```python
from build123d import *

# Parameters (mm, degrees)
SKETCH1_R      = 18
GEARBOX_DEPTH  = 42.5
SKETCH2_R      = 17
MOTOR_DEPTH    = 44.5
SKETCH3_R      = 11
PLATFORM_DEPTH = 2
SKETCH4_R      = 1.5
SCREWS_DEPTH   = 5


with BuildPart() as part:
    # Sketch1 → Gearbox (new body)
    with BuildSketch(Plane.XY):
        Circle(SKETCH1_R)
    extrude(amount=GEARBOX_DEPTH)

    # Sketch2 → Motor (add)
    with BuildSketch(Plane.XY.offset(42.5)):
        Circle(SKETCH2_R)
    extrude(amount=MOTOR_DEPTH)

    # Sketch3 → Platform (add)
    with BuildSketch(Plane(origin=(0, 0, 0), x_dir=(-1, 0, 0), z_dir=(0, 0, -1))):
        Circle(SKETCH3_R)
    extrude(amount=PLATFORM_DEPTH)

    # Sketch4 → Screws (cut)
    with BuildSketch(Plane(origin=(0, 0, 0), x_dir=(-1, 0, 0), z_dir=(0, 0, -1))):
        with Locations((0, 14)):
            Circle(SKETCH4_R)
        with Locations((14, 0)):
            Circle(SKETCH4_R)
        with Locations((0, -14)):
            Circle(SKETCH4_R)
        with Locations((-14, 0)):
            Circle(SKETCH4_R)
    extrude(amount=-SCREWS_DEPTH, mode=Mode.SUBTRACT)


solid = part.part
```
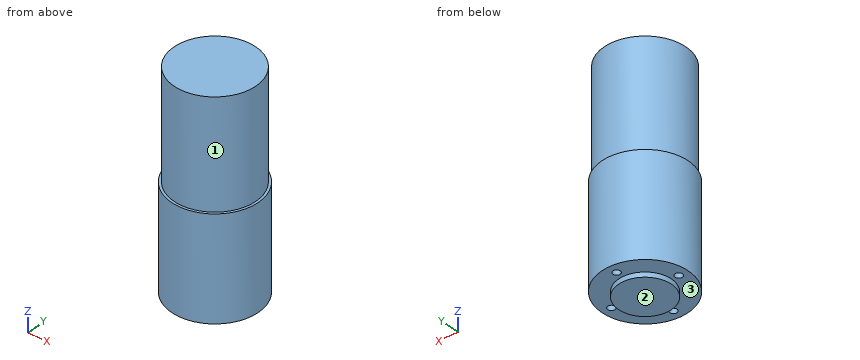
The listing builds one solid part. Answer for the finished solid, in the listing's coordinates (mm). Face numbers are marked on the shaded views. A direction names the side the tool comes from. Coordinates: 2 decimals unless noted, no trailing zeros. Order: outer loops, then holes, each group sorted by start corner. A loop starts at its lowest first (then second) coordinate and runs counter-clockwise, first axis right, second up. Notation, with made-up numbers: M -22.5,51.25 L 31.5,51.25 A25 cw 31.5,70.25 Z; hole C -16,-6 d9. An arc over 180 degrees is marked long. Answer as a JSON object with one key per item and string values. Group by question number.
1. Straight lines are drawn through the part: line 1 (Y direction, x = 0, z = 2.7); line 2 (X direction, y = -7, z = 59); line 3 (Y direction, x = 14, z = 2). For each, find the intervals that lie inside material, in ascending order.
2. Flat-ended cylindrical pins translate along their axes: P1, Ø2.5, axis at x = 14.5, y = -0.5, coming from the -Z side; P2, Ø5, axis at x = 11, z = 66, coming from the +Y side; P3, Ø0.9, axis at x = -0.5, y = -13.5, coming from the -Z side. Find the tip coordinate at first contact, or state that the pin passes through.
3. Section A-A on y = 0 is taken. Write down the section's boundary in (x, z), then the cut area to 3 significant figures.
4. Section D-D on x = 9 is taken. Write down the section's boundary in (y, z).
5. A tool of negligible diameter and unlimited length cuts with its end or side. For the marked faces 1, 2 and 3, from which of +Z, -Z, +X, -X, +Y, -Y can it reach the whole face along a straight path? Write none if from no direction.
6. Section C-C on z = 18.5 is taken. Write down the section's boundary in (x, y), then the cut area to 3 significant figures.
Values follow:
{
 "1": {"line 1": "-18 to -15.5, -12.5 to 12.5, 15.5 to 18", "line 2": "-15.49 to 15.49", "line 3": "-11.31 to -1.5, 1.5 to 11.31"},
 "2": {"P1": "z = 0", "P2": "y = 14.72", "P3": "z = 5"},
 "3": {"outline": "M -18,0 L -15.5,0 L -15.5,5 L -12.5,5 L -12.5,0 L -11,0 L -11,-2 L 11,-2 L 11,0 L 12.5,0 L 12.5,5 L 15.5,5 L 15.5,0 L 18,0 L 18,42.5 L 17,42.5 L 17,87 L -17,87 L -17,42.5 L -18,42.5 Z", "area": "3,060 mm2"},
 "4": {"outline": "M -15.59,0 L -6.32,0 L -6.32,-2 L 6.32,-2 L 6.32,0 L 15.59,0 L 15.59,42.5 L 14.42,42.5 L 14.42,87 L -14.42,87 L -14.42,42.5 L -15.59,42.5 Z"},
 "5": {"face 1": "+Z", "face 2": "-Z, +X, -X, +Y, -Y", "face 3": "-Z"},
 "6": {"outline": "C 0,0 d36", "area": "1,020 mm2"}
}
